Source: three-view drawing plus pictorial views. Frame: mm from the lowest corner of the part. Coordinates: 2 decimals unless noted, no trailing zeros. Write each loop counter-clockwise with the first axis right and the second up, starting at its lowest first coordinate (ties: lowest second). Pieces come first, ordered by that corner, then holes. Notation, with made-up numbers: (37.25, 4) -> (51.25, 4) arc R16 ccw to (51.25, 8) -> close; hole circle Ø10 at (54, 82.5). An arc over 180 degrees is marked (long way). One line per item, written item: value.
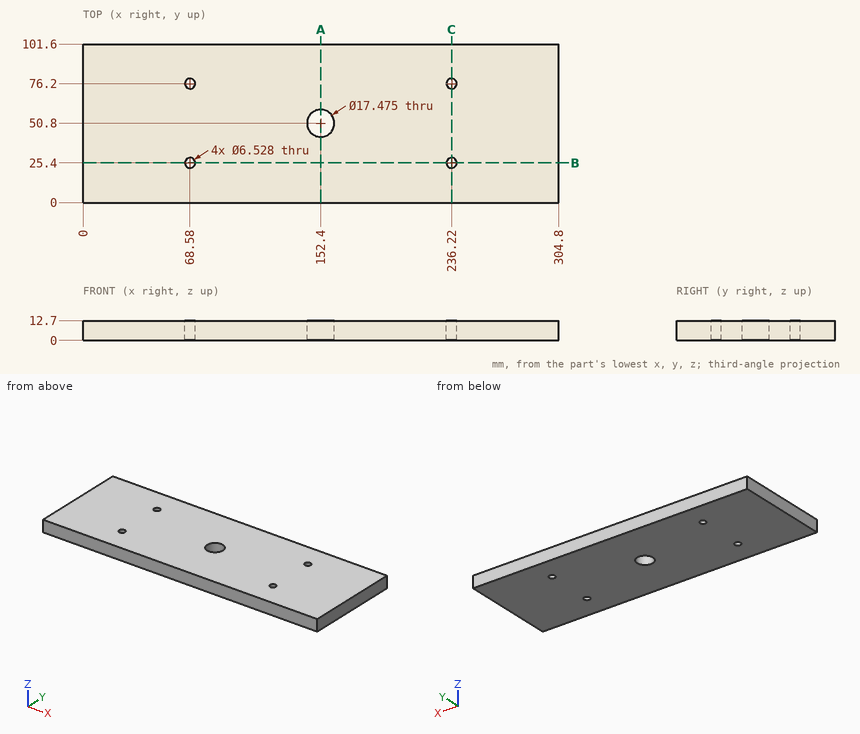
(1) Section B-B (y = 25.4). Return the cut outline in (x, z), then the cut area to 4 significant figures.
Responses:
outline: (0, 0) -> (65.32, 0) -> (65.32, 12.7) -> (0, 12.7) -> close; (71.84, 0) -> (232.96, 0) -> (232.96, 12.7) -> (71.84, 12.7) -> close; (239.48, 0) -> (304.8, 0) -> (304.8, 12.7) -> (239.48, 12.7) -> close
area: 3,705 mm2
(2) Line query: line 1 (X direction, y = 25.4, z = 3.5); line 2 (Y direction, x = 68.58, z = 7.25); line 3 (Y direction, x = 152.4, z = 3.5). Output: solid intervals per line, ascending. Write a range as [from, to].
Responses:
line 1: x = [0, 65.32], [71.84, 232.96], [239.48, 304.8]
line 2: y = [0, 22.14], [28.66, 72.94], [79.46, 101.6]
line 3: y = [0, 42.06], [59.54, 101.6]
(3) Section A-A (x = 152.4). Return the cut outline in (y, z), then the cut area to 3 significant figures.
Responses:
outline: (0, 0) -> (42.06, 0) -> (42.06, 12.7) -> (0, 12.7) -> close; (59.54, 0) -> (101.6, 0) -> (101.6, 12.7) -> (59.54, 12.7) -> close
area: 1,070 mm2
(4) First-contact query: pin 1 (5 mm diameter, centred on x = 68.58, y = 25.4, fed in from -Z). Flat tip, straight axial feed; report the tip coordinate or a pass-through.
Responses:
pin 1: passes through
(5) Section C-C (x = 236.22). Return the cut outline in (y, z).
Responses:
outline: (0, 0) -> (22.14, 0) -> (22.14, 12.7) -> (0, 12.7) -> close; (28.66, 0) -> (72.94, 0) -> (72.94, 12.7) -> (28.66, 12.7) -> close; (79.46, 0) -> (101.6, 0) -> (101.6, 12.7) -> (79.46, 12.7) -> close
